```python
from build123d import *

# Parameters (mm, degrees)
SKETCH2_W           = 70
SKETCH2_H           = 70
BOSS_EXTRUDE1_DEPTH = 20
FILLET1_R           = 10
HOLE1_D             = 10
HOLE1_DEPTH         = 20
HOLE2_D             = 12
CIRPATTERN1_COUNT   = 4


with BuildPart() as part:
    # Sketch1 → Revolve1 (revolve)
    with BuildSketch(Plane(origin=(0, 0, 0), x_dir=(1, 0, 0), z_dir=(0, 1, 0)), mode=Mode.PRIVATE) as revolve1_sk:
        Polygon((0, 15), (52, 15), (52, 39), (182, 39), (182, 69), (202, 69), (202, 24), (58, 24), (58, 9), (0, 9), align=None)
    revolve(revolve1_sk.sketch.rotate(Axis((0, 0, 0), (1, 0, 0)), 180), axis=Axis((0, 0, 0), (1, 0, 0)))

    # Sketch2 → Boss-Extrude1 (add)
    with BuildSketch(Plane.ZY):
        Rectangle(SKETCH2_W, SKETCH2_H)
    extrude(amount=BOSS_EXTRUDE1_DEPTH)

    # Fillet1
    fillet1_edges = [part.edges().sort_by_distance(p)[0] for p in [
        (-10, -35, 35),
        (-10, 35, 35),
        (-10, 35, -35),
        (-10, -35, -35),
    ]]
    fillet(fillet1_edges, radius=FILLET1_R)

    # Hole1
    with Locations(Plane.ZY.offset(20)):
        with Locations((25, 25), (25, -25), (-25, -25), (-25, 25)):
            Hole(HOLE1_D / 2, depth=HOLE1_DEPTH)

    # Hole2 (through all)
    with Locations(Plane.ZY.offset(-182)):
        with Locations((50, 0)):
            hole2 = Hole(HOLE2_D / 2)

    # CirPattern1: Hole2 ×4 about axis
    cirpattern1_axis = Axis((0, 0, 0), (1, 0, 0))
    for i in range(1, CIRPATTERN1_COUNT):
        add(hole2.rotate(cirpattern1_axis, i * 360 / CIRPATTERN1_COUNT), mode=Mode.SUBTRACT)


solid = part.part
```
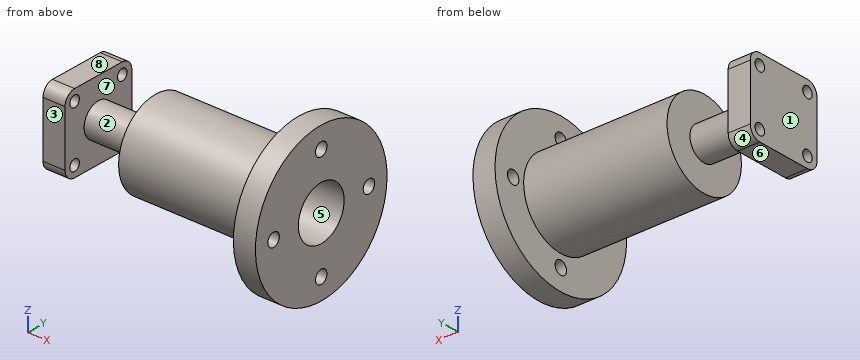
Could you check a few things on this model? Use its own coordinates, in mm. Face numbers are marked on the shaded views. A direction names the side the tool comes from. Round coordinates to 2 decimals unless told otherwise and drop trailing zeros. Order: outer loops, then holes, each group sorted by start corner. A loop starts at its lowest first (then second) coordinate and runs counter-clockwise, first axis right, second up. Notation, with made-up numbers: M 43,1.5 L 83,1.5 A25 cw 83,18.5 Z; hole C 27,60.5 d1. An arc over 180 degrees is marked long. One line per question, with ' | ' between items. Start each with the question number.
(1) Suppose I cut it at C-C on z = 50. List the corners of the cut face in (x, y) for me.
(2) For P1, Ø5, axis at x = 134.5, y = 21.5, coming from the -Z side; P2, Ø6, axis at x = -5.5, z = -2, coming from the +Y side; P3, Ø6, axis at x = 8, z = -13.5, coming from the -Y side, each with a flat end and sliding along its axis, tell me the tip position at first contact or that it passes through.
(3) Thinking about a two-plate mould opening in X: for the marked faces 1, 2 and 3, which applies, +X half, -X half, draft (parallel to the pull), parting line (faces both ways), or undercut?
(4) Suppose I cut it at D-D on x = 28. List the corners of the cut face in (y, z) for me.
(5) Please list where these lines run through material, in increasing order: line 1 along Y through (x, z) = (-8.25, -25); line 2 along X through (y, z) = (42.5, 33); line 3 along X through (y, z) = (9.5, 31.5).
(6) Suppose I cut it at A-A on y = 0. Count the separate pieces of the cut face and the enclosed holes in it, then the cut area to 3 significant figures.
(7) For the marked faces 4, 5, 6, 7 and 8, which set-ups out of +Z, -Z, +X, -X, +Y, -Y let a thin tool reach every point of the face, with its end or its side?
Geometry results:
1) outline: M 182,-47.55 L 202,-47.55 L 202,-6 L 182,-6 Z; M 182,6 L 202,6 L 202,47.55 L 182,47.55 Z
2) P1: z = -34.06 | P2: y = 35 | P3: y = -10.71
3) face 1: -X half | face 2: undercut | face 3: draft
4) outline: C 0,0 d30; hole C 0,0 d18
5) line 1: -35 to -30, -20 to 20, 30 to 35 | line 2: 182 to 202 | line 3: -20 to 0, 52 to 202
6) separate pieces: 3 | enclosed holes: 0 | area: 7,420 mm²
7) face 4: -Z, -X, +Y | face 5: +X | face 6: -Z, -X, +Y, -Y | face 7: none | face 8: +Z, -X, +Y, -Y
